from build123d import *

# Parameters (mm, degrees)
SKETCH1_R           = 2
BOSS_EXTRUDE1_DEPTH = 3
GROOVE_DEPTH        = 1


with BuildPart() as part:
    # Sketch1 → Boss-Extrude1 (new body)
    with BuildSketch(Plane.XY):
        with BuildLine():
            Line((163, 193), (-163, 193))
            Line((-163, 193), (-163, -190))
            Line((-163, -190), (-148, -190))
            Line((-148, -190), (-148, -173))
            Line((-148, -173), (-148, 168))
            ThreePointArc((-148, 168), (-145.071067812, 175.071067812), (-138, 178))
            Line((-138, 178), (138, 178))
            ThreePointArc((138, 178), (145.071067812, 175.071067812), (148, 168))
            Line((148, 168), (148, -173))
            Line((148, -173), (148, -190))
            Line((148, -190), (163, -190))
            Line((163, -190), (163, 193))
        make_face()
        with Locations((-157, -133)):
            Circle(SKETCH1_R, mode=Mode.SUBTRACT)
        with Locations((-157, -13)):
            Circle(SKETCH1_R, mode=Mode.SUBTRACT)
        with Locations((157, -133)):
            Circle(SKETCH1_R, mode=Mode.SUBTRACT)
        with Locations((157, -13)):
            Circle(SKETCH1_R, mode=Mode.SUBTRACT)
        with Locations((-157, 97)):
            Circle(SKETCH1_R, mode=Mode.SUBTRACT)
        with Locations((-157, 187)):
            Circle(SKETCH1_R, mode=Mode.SUBTRACT)
        with Locations((0, 187)):
            Circle(SKETCH1_R, mode=Mode.SUBTRACT)
        with Locations((157, 97)):
            Circle(SKETCH1_R, mode=Mode.SUBTRACT)
        with Locations((157, 187)):
            Circle(SKETCH1_R, mode=Mode.SUBTRACT)
    extrude(amount=BOSS_EXTRUDE1_DEPTH)

    # Sketch2 → Groove (cut)
    with BuildSketch(Plane.XY.offset(3)):
        Polygon((-152.5, -190), (-150.5, -190), (-150.5, 180.5), (150.5, 180.5), (150.5, -190), (152.5, -190), (152.5, 182.5), (-152.5, 182.5), align=None)
    extrude(amount=-GROOVE_DEPTH, mode=Mode.SUBTRACT)


solid = part.part
Could you check a few things on this model? Use its own coordinates, in mm. A direction names the side the tool comes from. Give positions to 0.01 mm unless a question says otherwise; leave off trailing zeros. Order: outer loops, then holes, each group sorted by start corner. A loop starts at its lowest first (then second) coordinate and runs counter-clockwise, first axis right, second up. Notation, with made-up numbers: (-9.5, -11.75) - (45.5, -11.75) arc R28 ccw to (45.5, 27.25) - close; hole circle Ø4 at (72, 6.5). An arc over 180 degrees is marked (long way). One line per item, written item: value. Start each with the question number.
1. Imagine slicing it at C-C on x = 12.5. List the corners of the cut face in (y, z) for me.
2. Imagine slicing it at A-A on y = 153. List the corners of the cut face in (x, z) for me, plus the area to 3 significant figures.
3. If I drill on probe 1 along X at (y, z) = (-26.5, 2.5); probe 2 along X at (y, z) = (-133, 2.3); probe 3 along Y at (x, z) = (-157, 1.05), over which ranges is the centre line in solid material (lowest first)?
4. Imagine slicing it at B-B on z = 1.3. Give the number of separate pieces and of enclosed holes in the cut face, plus the area to 3 significant figures.
5. For faces 3 (the face through (144.99, 175.15, 1.48)), 4 (the face through (-13, 187, 3)), which set-ups out of +Z, -Z, +X, -X, +Y, -Y let a thin tool reach every point of the face, with its end or its side?
6. Thinking about a two-plate mould opening in X: for faces 1 (the face through (-145.15, 174.99, 1.48)), 2 (the face through (-13, 187, 0)), which applies, +X half, -X half, draft (parallel to the pull), parting line (faces both ways), or undercut?
7. For P1, Ø0.5, axis at x = 65, z = 2.5, coming from the -Y side; P2, Ø6.5, axis at x = -157, y = -133, coming from the -Z side, each with a flat end and sliding along its axis, tell me the tip position at first contact or that it passes through.
Values:
1. outline: (178, 0) - (193, 0) - (193, 3) - (182.5, 3) - (182.5, 2) - (180.5, 2) - (180.5, 3) - (178, 3) - close
2. outline: (-163, 0) - (-148, 0) - (-148, 3) - (-150.5, 3) - (-150.5, 2) - (-152.5, 2) - (-152.5, 3) - (-163, 3) - close; (148, 0) - (163, 0) - (163, 3) - (152.5, 3) - (152.5, 2) - (150.5, 2) - (150.5, 3) - (148, 3) - close
2. area: 86.0 mm²
3. probe 1: -163 to -152.5, -150.5 to -148, 148 to 150.5, 152.5 to 163
3. probe 2: -163 to -159, -155 to -152.5, -150.5 to -148, 148 to 150.5, 152.5 to 155, 159 to 163
3. probe 3: -190 to -135, -131 to -15, -11 to 95, 99 to 185, 189 to 193
4. separate pieces: 1
4. enclosed holes: 9
4. area: 15,900 mm²
5. face 3: +Z, -Z, -Y
5. face 4: +Z, +X, -X, +Y, -Y
6. face 1: undercut
6. face 2: draft
7. P1: y = 178
7. P2: z = 0
